from build123d import *

# Parameters (mm, degrees)
SKETCH3_W                    = 131
SKETCH3_H                    = 54
BOSS_EXTRUDE2_DEPTH          = 5
F_3_0_3_DIAMETER_HOLE1_D     = 3
F_3_0_3_DIAMETER_HOLE1_DEPTH = 20
F_3_0_3_DIAMETER_HOLE1_TIP   = 0.901290929
SHELL1_T                     = -1.5
CUT_EXTRUDE1_DEPTH           = 114.452633288
FILLET2_START                = -28
FILLET2_DEPTH                = 120.497573337
FILLET2_2_ANGLE              = 180


with BuildPart() as part:
    # Sketch3 → Boss-Extrude2 (new body)
    with BuildSketch(Plane.XY):
        with BuildLine():
            Line((-65.5, 27), (65.5, 27))
            ThreePointArc((65.5, 27), (0, 92.5), (-65.5, 27))
        make_face()
        Rectangle(SKETCH3_W, SKETCH3_H)
    extrude(amount=BOSS_EXTRUDE2_DEPTH)

    # Ø3.0 (3) Diameter Hole1
    with Locations(Plane.XY.offset(5)):
        with Locations((-63.5, -17), (63.5, -17), (0, 89.5), (63.5, 31.210132452), (-63.5, 31.210132452)):
            Hole(F_3_0_3_DIAMETER_HOLE1_D / 2, depth=F_3_0_3_DIAMETER_HOLE1_DEPTH)
            with Locations((0, 0, -(F_3_0_3_DIAMETER_HOLE1_DEPTH + F_3_0_3_DIAMETER_HOLE1_TIP / 2))):  # 118° drill point
                Cone(0, F_3_0_3_DIAMETER_HOLE1_D / 2, F_3_0_3_DIAMETER_HOLE1_TIP, mode=Mode.SUBTRACT)

    # Shell1
    shell1_openings = [part.faces().sort_by_distance(p)[0] for p in [
        (0, 26.743328941, 5),
    ]]
    offset(amount=SHELL1_T, openings=shell1_openings)

    # Sketch6 → Cut-Extrude1 (cut, through all)
    with BuildSketch(Plane(origin=(0, 0, 0), x_dir=(-1, 0, 0), z_dir=(0, 0, -1))):
        with BuildLine():
            Line((-18, 27), (-18, -27))
            Line((-18, -27), (18, -27))
            Line((18, -27), (18, 27))
            ThreePointArc((18, 27), (0, 45), (-18, 27))
        make_face()
    extrude(amount=-CUT_EXTRUDE1_DEPTH, mode=Mode.SUBTRACT)

    # Fillet2: read off the stored shape, not the designer's step
    # Fillet2 outline → Fillet2 (cut)
    with BuildSketch(Plane(origin=(0, 0, 0), x_dir=(1, 0, 0), z_dir=(0, 1, 0)).offset(FILLET2_START)):
        with BuildLine():
            ThreePointArc((-65.5, -2.5), (-64.767766953, -0.732233047), (-63, 0))
            Line((-63, 0), (-65.5, 0))
            Line((-65.5, 0), (-65.5, -2.5))
        make_face()
        with BuildLine():
            ThreePointArc((63, 0), (64.767766953, -0.732233047), (65.5, -2.5))
            Line((65.5, -2.5), (65.5, 0))
            Line((65.5, 0), (63, 0))
        make_face()
    extrude(amount=FILLET2_DEPTH, mode=Mode.SUBTRACT)

    # Fillet2 2 outline → Fillet2 2 (revolve, cut)
    with BuildSketch(Plane.XZ.offset(-27)):
        with BuildLine():
            ThreePointArc((65.5, 2.5), (64.767766953, 0.732233047), (63, 0))
            Line((63, 0), (65.5, 0))
            Line((65.5, 0), (65.5, 2.5))
        make_face()
    revolve(axis=Axis((0, 27, 0), (0, 0, 1)), revolution_arc=FILLET2_2_ANGLE, mode=Mode.SUBTRACT)


solid = part.part
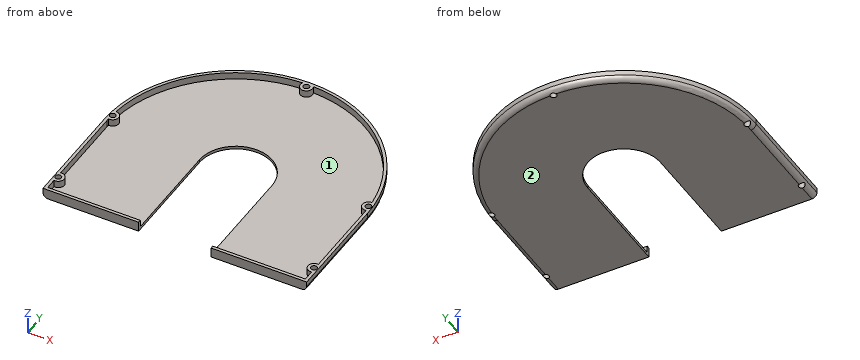
Verification items for the finished model (mm, model axes). Face numbers are marked on the shaded views. Coordinates: 2 decimals unless noted, no trailing zeros. Loops run counter-clockwise (first coordinate to the right, second up) from the corner with the lowest first, then second, coordinate; pieces in that order, holes last. Notation, with made-up numbers: (31.5, -7.5) -> (78.5, -7.5) arc R28 ccw to (78.5, 11.5) -> close; hole circle Ø7 at (85.5, -28). An arc over 180 degrees is marked (long way). Write each question's results on one line, items separated by ' | '.
Item 1: Gauge pin test, flat ends, axial feed: pin 1 (1.8 mm diameter, centred on x = -48.5, z = 3.5, fed in from +Y); pin 2 (1.5 mm diameter, centred on x = 37, z = 4, fed in from +Y); pin 3 (2.5 mm diameter, centred on x = 0, y = 89.5, fed in from +Z); pin 4 (1 mm diameter, centred on x = 39.5, z = 2.5, fed in from +Y). Record the tip position at first contact, or that the pin passes through.
Found:
pin 1: stops at y = 71.99 | pin 2: stops at y = 81.55 | pin 3: passes through | pin 4: stops at y = 79.62
Item 2: Material ranges on L1, parallel to X at y = -3, z = 3.55; L2, parallel to Z at x = -18.5, y = 52; L3, parallel to X at y = 35, z = 2.8, recorded low to high.
Found:
L1: x = -65.5 to -64, 64 to 65.5 | L2: z = 0 to 1.5 | L3: x = -65.01 to -63.5, 63.5 to 65.01
Item 3: Section check A-A, the plane y = 10. Enter the section's corners in (x, z).
Found:
outline: (-65.5, 2.5) arc R2.5 ccw to (-63, 0) -> (-18, 0) -> (-18, 1.5) -> (-64, 1.5) -> (-64, 5) -> (-65.5, 5) -> close; (18, 0) -> (63, 0) arc R2.5 ccw to (65.5, 2.5) -> (65.5, 5) -> (64, 5) -> (64, 1.5) -> (18, 1.5) -> close
Item 4: Section check B-B, the plane x = 0. Enter the section's corners in (y, z).
Found:
outline: (45, 0) -> (88, 0) -> (88, 5) -> (86.5, 5) -> (86.5, 1.5) -> (45, 1.5) -> close; (91, 0.21) arc R2.5 ccw to (92.5, 2.5) -> (92.5, 5) -> (91, 5) -> close
Item 5: Mould release check, pull along Y, two halves, no side actions. Record for the marked faces 1 and 2: +Y half, -Y half, draft (parallel to the pull), parting line (faces both ways), or undercut.
Found:
face 1: undercut | face 2: draft
